from build123d import *

# Parameters (mm, degrees)
BOX_W        = 26
BOX_H        = 571
BOX_DEPTH    = 196
POCKET_DEPTH = 26.001


with BuildPart() as part:
    # Box → Box (new body)
    with BuildSketch(Plane.XY):
        with Locations((13, 285.5)):
            Rectangle(BOX_W, BOX_H)
    extrude(amount=BOX_DEPTH)

    # Sketch (on Face1 of Box) → Pocket (cut, through all)
    with BuildSketch(Plane(origin=(0, 0, 0), x_dir=(0, -1, 0), z_dir=(-1, 0, 0))):
        with BuildLine():
            ThreePointArc((-170, 176), (-152.426407, 133.573593), (-110, 116))
            Line((-110, 116), (0, 116))
            Line((0, 200), (0, 116))
            Line((-170, 200), (0, 200))
            Line((-170, 200), (-170, 176))
        make_face()
    extrude(amount=-POCKET_DEPTH, mode=Mode.SUBTRACT)


solid = part.part
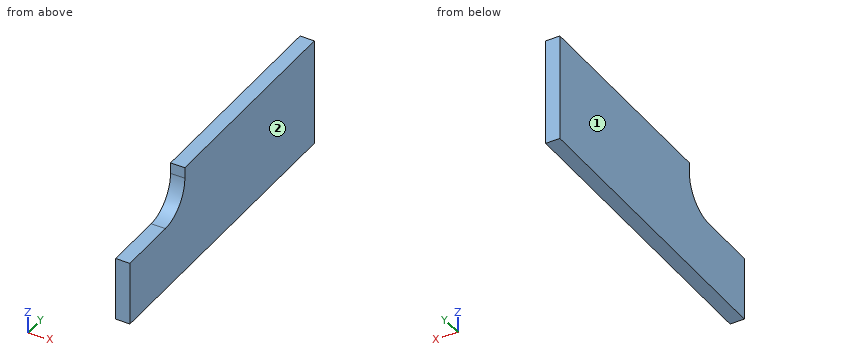
The listing builds one solid part. Answer for the finished solid, in the listing's coordinates (mm). Face numbers are marked on the shaded views. Coordinates: 2 decimals unless noted, no trailing zeros. Loops run counter-clockwise (first coordinate to the right, second up) from the corner with the lowest first, then second, coordinate; pieces in that order, holes last. Notation, with made-up numbers: (-23.75, -36.5) -> (9.25, -36.5) arc R12 ccw to (9.25, -30.5) -> close; hole circle Ø11 at (-2, 52). An arc over 180 degrees is marked (long way). Write item = value, one per line. Start each with the question number.
1) Straight lines are drawn through the part: line 1 (Z direction, x = 22, y = 91.5); line 2 (Y direction, x = 15.25, z = 186); line 3 (Y direction, x = 20.5, z = 150). For each, find the intervals that lie inside material, in ascending order. Write a range as from..to.
2) A cutting plane is placed at B-B (z = 161). Give the vertices of the cut face in (x, y), then the cut area to 3 significant figures.
3) The mould has two halves that part along X. Classify the marked faces 1 and 2: released by +X, released by -X, zero draft, split by the parting line, or undercut.
4) A cutting plane is placed at C-C (y = 89). Give the vertices of the cut face in (x, z).
5) A cutting plane is placed at A-A (x = 20.25). Give the vertices of the cut face in (y, z).
6) Given pin 1 Ø2 at (x, y) = (4.5, 101) entering from +Z; pin 2 Ø1.5 at (x, y) = (19.5, 140) entering from +Z; pin 3 Ø4 at (x, z) = (10.5, 156.5) entering from -Y, each flat-ended and moving along its own axis, determine where each tip first touches the part or whether it passes through.
Responses:
q1.line_1 = 0..116
q1.line_2 = 170..571
q1.line_3 = 164.07..571
q2.outline = (0, 168.09) -> (26, 168.09) -> (26, 571) -> (0, 571) -> close
q2.area = 10,500 mm²
q3.face_1 = released by -X
q3.face_2 = released by +X
q4.outline = (0, 0) -> (26, 0) -> (26, 116) -> (0, 116) -> close
q5.outline = (0, 0) -> (571, 0) -> (571, 196) -> (170, 196) -> (170, 176) arc R60 cw to (110, 116) -> (0, 116) -> close
q6.pin_1 = 116
q6.pin_2 = 124.48
q6.pin_3 = 166.02
